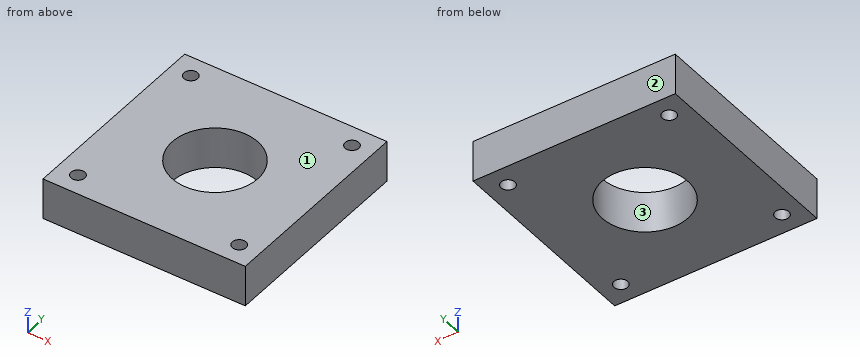
```python
from build123d import *

# Parameters (mm, degrees)
SKETCH1_W               = 59
SKETCH1_H               = 59
BOSS_EXTRUDE1_DEPTH     = 12
CUT_EXTRUDE1_REACH      = 45.411
SKETCH2_R               = 2
MIRROR2_COPY_1_REACH    = 45.411
MIRROR2_COPY_1_SKETCH_R = 2
CUT_EXTRUDE2_REACH      = 45.411
SKETCH3_R               = 12.5


with BuildPart() as part:
    # Sketch1 → Boss-Extrude1 (new body)
    with BuildSketch(Plane.XY):
        Rectangle(SKETCH1_W, SKETCH1_H)
    extrude(amount=BOSS_EXTRUDE1_DEPTH)

    # Sketch2 → Cut-Extrude1 (cut, up to next)
    with BuildSketch(Plane.XY.offset(12), mode=Mode.PRIVATE) as cut_extrude1_sk1:
        with Locations((-23.5, 23.5)):
            Circle(SKETCH2_R)
    cut_extrude1_tool1 = extrude(cut_extrude1_sk1.sketch, amount=-CUT_EXTRUDE1_REACH, mode=Mode.PRIVATE) & part.part
    cut_extrude1 = cut_extrude1_tool1.solids().sort_by_distance((-23.5, 23.5, 12))[0]
    add(cut_extrude1, mode=Mode.SUBTRACT)

    # Mirror1: Cut-Extrude1 across plane
    add(cut_extrude1.mirror(Plane(origin=(0, 0, 0), x_dir=(0, 0, 1), z_dir=(1, 0, 0))), mode=Mode.SUBTRACT)

    # Mirror2: Cut-Extrude1 across plane
    add(cut_extrude1.mirror(Plane.ZX), mode=Mode.SUBTRACT)

    # Mirror2 copy 1 sketch → Mirror2 copy 1 (cut, up to next)
    with BuildSketch(Plane(origin=(0, 0, 12), x_dir=(-1, 0, 0), z_dir=(0, 0, 1)), mode=Mode.PRIVATE) as mirror2_copy_1_sk1:
        with Locations((-23.5, 23.5)):
            Circle(MIRROR2_COPY_1_SKETCH_R)
    mirror2_copy_1_tool1 = extrude(mirror2_copy_1_sk1.sketch, amount=-MIRROR2_COPY_1_REACH, mode=Mode.PRIVATE) & part.part
    add(mirror2_copy_1_tool1.solids().sort_by_distance((23.5, -23.5, 12))[0], mode=Mode.SUBTRACT)

    # Sketch3 → Cut-Extrude2 (cut, up to next)
    with BuildSketch(Plane.XY.offset(12), mode=Mode.PRIVATE) as cut_extrude2_sk1:
        Circle(SKETCH3_R)
    cut_extrude2_tool1 = extrude(cut_extrude2_sk1.sketch, amount=-CUT_EXTRUDE2_REACH, mode=Mode.PRIVATE) & part.part
    add(cut_extrude2_tool1.solids().sort_by_distance((0, 0, 12))[0], mode=Mode.SUBTRACT)


solid = part.part
```
CAD build for the part. Positions are in the model's coordinates, mm. Face numbers are marked on the shaded views. Coordinates: 2 decimals unless noted, no trailing zeros. Order: outer loops, then holes, each group sorted by start corner. A loop starts at its lowest first (then second) coordinate and runs counter-clockwise, first axis right, second up. Notation, with made-up numbers: (-6, -38.75) - (10, -38.75) arc R21 cw to (10, -20.75) - close; hole circle Ø6 at (80.5, -11). An arc over 180 degrees is marked (long way). Answer in a Markdown table with one row per item.
1. Slice it at B-B, the plane z = 1.75. List the corners of the cut face in (x, y).
Answer:
| item | result |
|---|---|
| outline | (-29.5, -29.5) - (29.5, -29.5) - (29.5, 29.5) - (-29.5, 29.5) - close; hole circle Ø4 at (-23.5, -23.5); hole circle Ø4 at (-23.5, 23.5); hole circle Ø25 at (0, 0); hole circle Ø4 at (23.5, -23.5); hole circle Ø4 at (23.5, 23.5) |
2. Pull direction Y, two halves, no side cores. Call the marked faces 1, 2 and 3: +Y half, -Y half, draft (parallel to the pull), parting line (faces both ways), or undercut.
Answer:
| item | result |
|---|---|
| face 1 | draft |
| face 2 | +Y half |
| face 3 | undercut |
3. Slice it at D-D, the plane x = 0. List the corners of the cut face in (y, z), then the cut area to 3 significant figures.
Answer:
| item | result |
|---|---|
| outline | (-29.5, 0) - (-12.5, 0) - (-12.5, 12) - (-29.5, 12) - close; (12.5, 0) - (29.5, 0) - (29.5, 12) - (12.5, 12) - close |
| area | 408 mm² |
4. Drill centre lines: L1, parallel to Y at x = 23.5, z = 3.75; L2, parallel to Y at x = 0, z = 2.5; L3, parallel to Y at x = -25, z = 3.25. Where is each one in solid material? Low to high. Write a range as from..to.
Answer:
| item | result |
|---|---|
| L1 | -29.5..-25.5, -21.5..21.5, 25.5..29.5 |
| L2 | -29.5..-12.5, 12.5..29.5 |
| L3 | -29.5..-24.82, -22.18..22.18, 24.82..29.5 |
5. Flat gauge pin, fed straight in: P1, Ø3.5, axis at x = 23.5, y = 23.5, coming from the +Z side. Where does the tip first touch, or does it go through?
Answer:
| item | result |
|---|---|
| P1 | through |
6. Slice it at A-A, the plane x = 23.5. List the corners of the cut face in (y, z), then the cut area to 3 significant figures.
Answer:
| item | result |
|---|---|
| outline | (-29.5, 0) - (-25.5, 0) - (-25.5, 12) - (-29.5, 12) - close; (-21.5, 0) - (21.5, 0) - (21.5, 12) - (-21.5, 12) - close; (25.5, 0) - (29.5, 0) - (29.5, 12) - (25.5, 12) - close |
| area | 612 mm² |
